Geometry check sheet. Reference: the model listing, model coordinates, mm. Coordinates: 2 decimals unless noted, no trailing zeros. Order: outer loops, then holes, each group sorted by start corner. A loop starts at its lowest first (then second) coordinate and runs counter-clockwise, first axis right, second up. Notation, with made-up numbers: (-27, 20) - (-21, 20) arc R27 ccw to (-21, 48) - close; hole circle Ø3 at (-9, 40). An arc over 180 degrees is marked (long way). Use CSV: the item, a comma, the result in double quotes. Start each with the question number.
1) Sectioned sample at A-A, the plane z = 47. Record the cut outline in (x, y), and give its area (3 significant figures).
2) Thickness scan on probe 1 along X at (y, z) = (12.5, 5.25); probe 2 along Z at (x, y) = (-30.75, 10); probe 3 along X at (y, z) = (13.75, 5.5). Record the ranges inside material, lowest first. Write a range as [from, to].
3) Depth check by flat-ended pin: P1, Ø3.5, axis at x = 80, y = 12.5, coming from the -Z side; P2, Ø2.5, axis at x = 100, y = 12.5, coming from the +Z side; P3, Ø4, axis at x = 40, y = 12.5, coming from the +Z side. Enter the tip coordinate at first touch or a pass-through.
from build123d import *

# Parameters (mm, degrees)
BOSS_EXTRUDE1_DEPTH        = 55
SKETCH2_W                  = 5
SKETCH2_H                  = 70
BOSS_EXTRUDE2_DEPTH        = 5
M5_TAPPED_HOLE1_AT_2_COUNT = 2
M5_TAPPED_HOLE1_AT_2_PITCH = 20
M5_TAPPED_HOLE1_AT_3_COUNT = 2
M5_TAPPED_HOLE1_AT_3_PITCH = 40
M5_TAPPED_HOLE1_AT_4_COUNT = 2
M5_TAPPED_HOLE1_AT_4_PITCH = 60
M5_TAPPED_HOLE1_AT_5_COUNT = 2
M5_TAPPED_HOLE1_AT_5_PITCH = 80
CUT_EXTRUDE1_DEPTH         = 126
SKETCH9_W                  = 55
SKETCH9_H                  = 20
BOSS_EXTRUDE3_DEPTH        = 5
CHAMFER1_SIZE              = 1.5
BOSS_EXTRUDE4_DEPTH        = 50
M6_TAPPED_HOLE2_D          = 5
M6_TAPPED_HOLE2_DEPTH      = 23.497848452
M6_TAPPED_HOLE2_TIP        = 1.502151548


with BuildPart() as part:
    # Sketch1 → Boss-Extrude1 (new body)
    with BuildSketch(Plane.XY):
        Polygon((0, 0), (110, 0), (110, 20), (20, 20), (20, 70), (0, 70), align=None)
    extrude(amount=BOSS_EXTRUDE1_DEPTH)

    # Sketch2 → Boss-Extrude2 (add)
    with BuildSketch(Plane.ZY):
        with Locations((52.5, 35)):
            Rectangle(SKETCH2_W, SKETCH2_H)
        with Locations((2.5, 35)):
            Rectangle(SKETCH2_W, SKETCH2_H)
    extrude(amount=BOSS_EXTRUDE2_DEPTH)

    # Sketch4 → M5 Tapped Hole1 (revolve, cut)
    with BuildSketch(Plane(origin=(100, 12.5, 55), x_dir=(0, -1, 0), z_dir=(1, 0, 0))):
        Polygon((0, 0), (0, 15.2618073), (2.1, 14), (2.1, 0), align=None)
    m5_tapped_hole1 = revolve(axis=Axis((100, 12.5, 61.35), (0, 0, -1)), mode=Mode.SUBTRACT)

    # M5 Tapped Hole1 at 2: M5 Tapped Hole1 ×2
    with Locations(*[(-i * M5_TAPPED_HOLE1_AT_2_PITCH, 0, 0) for i in range(1, M5_TAPPED_HOLE1_AT_2_COUNT)]):
        add(m5_tapped_hole1, mode=Mode.SUBTRACT)

    # M5 Tapped Hole1 at 3: M5 Tapped Hole1 ×2
    with Locations(*[(-i * M5_TAPPED_HOLE1_AT_3_PITCH, 0, 0) for i in range(1, M5_TAPPED_HOLE1_AT_3_COUNT)]):
        add(m5_tapped_hole1, mode=Mode.SUBTRACT)

    # M5 Tapped Hole1 at 4: M5 Tapped Hole1 ×2
    with Locations(*[(-i * M5_TAPPED_HOLE1_AT_4_PITCH, 0, 0) for i in range(1, M5_TAPPED_HOLE1_AT_4_COUNT)]):
        add(m5_tapped_hole1, mode=Mode.SUBTRACT)

    # M5 Tapped Hole1 at 5: M5 Tapped Hole1 ×2
    with Locations(*[(-i * M5_TAPPED_HOLE1_AT_5_PITCH, 0, 0) for i in range(1, M5_TAPPED_HOLE1_AT_5_COUNT)]):
        add(m5_tapped_hole1, mode=Mode.SUBTRACT)

    # Mirror1: M5 Tapped Hole1 across plane
    add(m5_tapped_hole1.mirror(Plane.XY.offset(27.5)), mode=Mode.SUBTRACT)

    # Mirror1 copy 1 sketch → Mirror1 copy 1 (revolve, cut)
    with BuildSketch(Plane(origin=(80, 12.5, 0), x_dir=(0, -1, 0), z_dir=(1, 0, 0))):
        Polygon((0, 0), (0, -15.2618073), (2.1, -14), (2.1, 0), align=None)
    revolve(axis=Axis((80, 12.5, -6.35), (0, 0, -1)), mode=Mode.SUBTRACT)

    # Mirror1 copy 2 sketch → Mirror1 copy 2 (revolve, cut)
    with BuildSketch(Plane(origin=(60, 12.5, 0), x_dir=(0, -1, 0), z_dir=(1, 0, 0))):
        Polygon((0, 0), (0, -15.2618073), (2.1, -14), (2.1, 0), align=None)
    revolve(axis=Axis((60, 12.5, -6.35), (0, 0, -1)), mode=Mode.SUBTRACT)

    # Mirror1 copy 3 sketch → Mirror1 copy 3 (revolve, cut)
    with BuildSketch(Plane(origin=(40, 12.5, 0), x_dir=(0, -1, 0), z_dir=(1, 0, 0))):
        Polygon((0, 0), (0, -15.2618073), (2.1, -14), (2.1, 0), align=None)
    revolve(axis=Axis((40, 12.5, -6.35), (0, 0, -1)), mode=Mode.SUBTRACT)

    # Mirror1 copy 4 sketch → Mirror1 copy 4 (revolve, cut)
    with BuildSketch(Plane(origin=(20, 12.5, 0), x_dir=(0, -1, 0), z_dir=(1, 0, 0))):
        Polygon((0, 0), (0, -15.2618073), (2.1, -14), (2.1, 0), align=None)
    revolve(axis=Axis((20, 12.5, -6.35), (0, 0, -1)), mode=Mode.SUBTRACT)

    # Sketch8 → Cut-Extrude1 (cut)
    with BuildSketch(Plane.XY.offset(55)):
        Polygon((17, 20), (17, 0), (-5, 0), (-5, 70), (20, 70), (20, 20), align=None)
    extrude(amount=-CUT_EXTRUDE1_DEPTH, mode=Mode.SUBTRACT)

    # Sketch9 → Boss-Extrude3 (add)
    with BuildSketch(Plane.ZY.offset(-17)):
        with Locations((27.5, 10)):
            Rectangle(SKETCH9_W, SKETCH9_H)
    extrude(amount=BOSS_EXTRUDE3_DEPTH)

    # Chamfer1
    chamfer1_edges = [part.edges().sort_by_distance(p)[0] for p in [
        (110, 20, 27.5),
        (110, 0, 27.5),
        (110, 10, 55),
        (61, 20, 55),
        (61, 20, 0),
        (110, 10, 0),
        (61, 0, 0),
        (61, 0, 55),
    ]]
    chamfer(chamfer1_edges, length=CHAMFER1_SIZE)

    # Sketch10 → Boss-Extrude4 (add)
    with BuildSketch(Plane.ZY.offset(-12)):
        Polygon((0, 18.5), (1.5, 20), (53.5, 20), (55, 18.5), (55, 1.5), (53.5, 0), (1.5, 0), (0, 1.5), align=None)
    extrude(amount=BOSS_EXTRUDE4_DEPTH)

    # M6 Tapped Hole2
    with Locations(Plane.ZY.offset(38)):
        with Locations((15, 10), (40, 10)):
            Hole(M6_TAPPED_HOLE2_D / 2, depth=M6_TAPPED_HOLE2_DEPTH)
            with Locations((0, 0, -(M6_TAPPED_HOLE2_DEPTH + M6_TAPPED_HOLE2_TIP / 2))):  # 118° drill point
                Cone(0, M6_TAPPED_HOLE2_D / 2, M6_TAPPED_HOLE2_TIP, mode=Mode.SUBTRACT)


solid = part.part
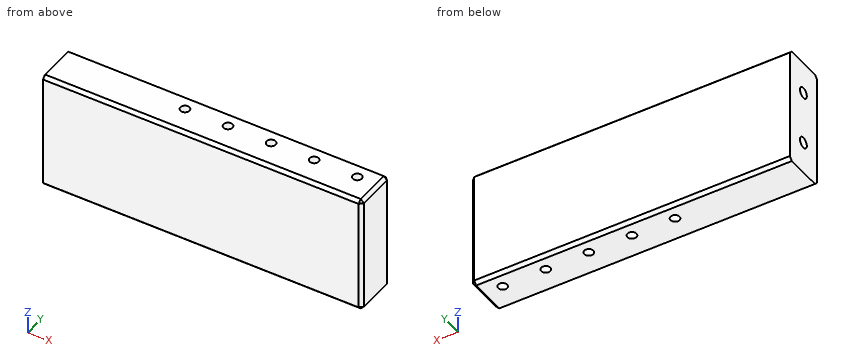
Evaluation:
1,outline,"(-38, 0) - (108.5, 0) - (110, 1.5) - (110, 18.5) - (108.5, 20) - (-38, 20) - close; hole circle Ø4.2 at (20, 12.5); hole circle Ø4.2 at (40, 12.5); hole circle Ø4.2 at (60, 12.5); hole circle Ø4.2 at (80, 12.5); hole circle Ø4.2 at (100, 12.5)"
1,area,"2,890 mm²"
2,probe 1,"[-38, 17.9], [22.1, 37.9], [42.1, 57.9], [62.1, 77.9], [82.1, 97.9], [102.1, 110]"
2,probe 2,"[0, 12.5], [17.5, 37.5], [42.5, 55]"
2,probe 3,"[-38, 18.31], [21.69, 38.31], [41.69, 58.31], [61.69, 78.31], [81.69, 98.31], [101.69, 110]"
3,P1,"z = 14.21"
3,P2,"z = 40.49"
3,P3,"z = 40.94"
